Autodesk Inventor part; units mm, degrees
ref_plane "Work Plane1" through (-25.4, 0, 0) normal (1, 0, 0) x (0, 1, 0)
ref_plane "XZ Plane" through (0, 0, 0) normal (0, 1, 0) x (-1, 0, 0)
ref_plane "XY Plane" through (0, 0, 0) normal (0, 0, 1) x (1, 0, 0)
sketch "Sketch1" plane through (0, 0, 0) normal (0, 1, 0) x (-1, 0, 0)
  line L0 (0, 0) -> (50.8, 0)
  line L1 (50.8, 0) -> (50.8, -203.2)
  line L2 (50.8, -203.2) -> (0, -203.2)
  line L3 (0, -203.2) -> (0, 0)
  dimension "d0" = 50.8
  dimension "d1" = 203.2
extrude "Extrusion1" add sketch "Sketch1" along normal blind 508
fillet "Fillet1" radius 25.4 1 edges at (0, 254, 0)
fillet "Fillet2" radius 25.4 1 edges at (0, 254, -203.2)
ref_plane "Work Plane1" through (-25.4, 0, 0) normal (1, 0, 0) x (0, 1, 0)
properties part number "SailPost-ver2-1111-2021"
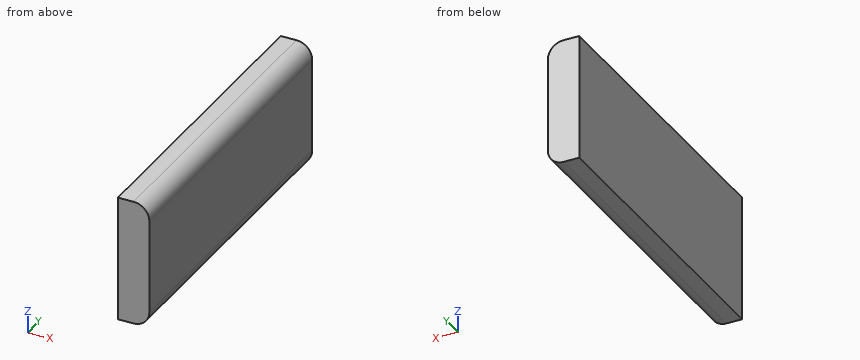
Input: part model. Units: mm. Frame: model coordinates. Coordinates: 2 decimals unless noted, no trailing zeros. Write each loop counter-clockwise with the first axis right and the second up, starting at its lowest first coordinate (ties: lowest second). Pieces come first, ordered by that corner, then holes. Notation, with made-up numbers: (-9, 0) -> (9, 0) arc R24 ccw to (9, 32) -> close; hole circle Ø11 at (-38, -16). An arc over 180 degrees is marked (long way). Write each question's results on one line, items separated by ' | '.
Item 1: Material intervals for probe 1 along Z at (x, y) = (-9.5, 261); probe 2 along Z at (x, y) = (-20.5, 258); probe 3 along X at (y, z) = (116.5, -186), sorted ascending.
Conclusion:
probe 1: z = -197.61 to -5.59 | probe 2: z = -202.72 to -0.48 | probe 3: x = -50.8 to -1.36
Item 2: Section query C-C on x = -16. Return loops of the section in (y, z).
Conclusion:
outline: (0, -201.4) -> (508, -201.4) -> (508, -1.8) -> (0, -1.8) -> close
Item 3: Section query B-B on z = -19. Return loops of the section in (x, y), plus the area to 3 significant figures.
Conclusion:
outline: (-50.8, 0) -> (-0.82, 0) -> (-0.82, 508) -> (-50.8, 508) -> close | area: 25,400 mm^2
Item 4: Section query A-A on y = 36. Return loops of the section in (x, z).
Conclusion:
outline: (-50.8, -203.2) -> (-25.4, -203.2) arc R25.4 ccw to (0, -177.8) -> (0, -25.4) arc R25.4 ccw to (-25.4, 0) -> (-50.8, 0) -> close
Item 5: Pin query (flat end, axial travel): pin 1 Ø5 at (x, y) = (-10.5, 350) entering from -Z; pin 2 Ø6 at (x, y) = (-15, 116) entering from -Z. Return the tip coordinate at first contact, or that it passes through.
Conclusion:
pin 1: stops at z = -199.97 | pin 2: stops at z = -202.1
